Autodesk Fusion 360 part; units mm, degrees
sketch "Sketch1" plane through (0, 0, 0) normal (0, 0, 1) x (1, 0, 0)
  circle A0 centre (0, 0) radius 4
  line L0 (0, 0) -> (-60.5, 0) construction
  line L1 (-60.5, 0) -> (-121, 0) construction
  circle A1 centre (-60.5, 0) radius 3.15
  circle A2 centre (-121, 0) radius 3.15
  circle A3 centre (-60.5, 0) radius 47 construction
  circle A4 centre (-121, 0) radius 47 construction
  circle A5 centre (0, 0) radius 17.5
  circle A6 centre (-60.5, 0) radius 17 construction
  circle A7 centre (0, 0) radius 12.5 construction
  circle A8 centre (0, 30) radius 2.25
  circle A9 centre (0, -30) radius 2.25
  circle A10 centre (0, 30) radius 6 construction
  circle A11 centre (0, -30) radius 6 construction
  line L2 (-90.75, 0) -> (-90.75, 50) construction
  circle A12 centre (-90.75, 50) radius 7.5
  circle A13 centre (-90.75, 50) radius 2.25
  line L3 (-90.75, 0) -> (-90.75, -50) construction
  circle A14 centre (-90.75, -50) radius 7.5
  circle A15 centre (-90.75, -50) radius 2.25
  line L4 (-121, 0) -> (-151.25, 0) construction
  line L5 (-151.25, 0) -> (-151.25, 50) construction
  circle A16 centre (-151.25, 50) radius 7.5
  circle A17 centre (-151.25, 50) radius 2.25
  line L6 (-151.25, 0) -> (-151.25, -50) construction
  circle A18 centre (-151.25, -50) radius 7.5
  circle A19 centre (-151.25, -50) radius 2.25
  circle A20 centre (-20, 40) radius 7.5
  line L7 (-20, 40) -> (-20, 0) construction
  line L8 (-20, 0) -> (-20, -40) construction
  circle A21 centre (-20, -40) radius 7.5
  circle A22 centre (-20, -40) radius 2.25
  circle A23 centre (-20, 40) radius 2.25
  line L9 (-89.7004, -57.4262) -> (-18.9504, -47.4262)
  circle A24 centre (0, -30) radius 7.5
  circle A25 centre (0, 30) radius 7.5
  line L10 (-89.7004, 57.4262) -> (-18.9504, 47.4262)
  circle A26 centre (-196.5959, 0) radius 60
  line L11 (-16.6459, 46.7082) -> (3.3541, 36.7082)
  line L12 (7.0711, 32.5) -> (16.4992, 5.8333)
  line L13 (7.0711, -32.5) -> (16.4992, -5.8333)
  line L14 (-16.6459, -46.7082) -> (3.3541, -36.7082)
  circle A27 centre (-121, 86.6222) radius 40
  line L15 (-151.25, -57.5) -> (-90.75, -57.5)
  line L16 (-160.1233, -61.9813) -> (16.4992, -61.9813) construction
  circle A28 centre (0, 0) radius 8.5 construction
  circle A29 centre (0, 8.5) radius 1.4
  circle A30 centre (0, -8.5) radius 1.4
  line L17 (-151.25, 57.5) -> (-90.75, 57.5)
  dimension "d1" = 8
  dimension "d2" = 60.5
  dimension "d4" = 60.5
  dimension "d6" = 6.3
  dimension "d7" = 6.3
  dimension "d8" = 94
  dimension "d9" = 94
  dimension "d10" = 35
  dimension "d11" = 34
  dimension "d12" = 25
  dimension "d13" = 4.5
  dimension "d14" = 4.5
  dimension "d15" = 60
  dimension "d16" = 12
  dimension "d17" = 12
  dimension "d18" = 15
  dimension "d19" = 50
  dimension "d20" = 4.5
  dimension "d21" = 15
  dimension "d22" = 4.5
  dimension "d23" = 30.25
  dimension "d24" = 15
  dimension "d25" = 4.5
  dimension "d26" = 15
  dimension "d27" = 4.5
  dimension "d28" = 15
  dimension "d29" = 40
  dimension "d30" = 20
  dimension "d31" = 15
  dimension "d32" = 4.5
  dimension "d33" = 4.5
  dimension "d34" = 15
  dimension "d35" = 15
  dimension "d36" = 120
  dimension "d37" = 80
  dimension "d44" = 17
  dimension "d45" = 2.8
  dimension "d46" = 2.8
extrude "Extrude1" add sketch "Sketch1" along normal blind 3.175 contours A5 | A5 A12 A14 A16 A18 A20 A21 L9 A24 A25 L10 A26 L11 L12 L13 L14 A27 L15 | A25 | A24 | A20 | A21 | A12 | A14 | A18 | A16
ref_plane "WorkPlane1" through (-70.7689, 0, 3.175) normal (0, 0, 1) x (1, 0, 0)
sketch "Sketch2" plane through (0, 0, 3.175) normal (0, 0, 1) x (1, 0, 0)
  circle A0 centre (-90.75, -50) radius 2.25
  circle A1 centre (0, 30) radius 2.25
  circle A2 centre (-151.25, -50) radius 2.25
  circle A3 centre (0, -30) radius 2.25
  circle A4 centre (0, 0) radius 4
  circle A5 centre (0, 8.5) radius 1.4
  circle A6 centre (0, -8.5) radius 1.4
  circle A7 centre (-20, -40) radius 2.25
  circle A8 centre (-90.75, 50) radius 2.25
  circle A9 centre (-20, 40) radius 2.25
  circle A10 centre (-151.25, 50) radius 2.25
  circle A11 centre (-60.5, 0) radius 3.15
  circle A12 centre (-121, 0) radius 3.15
  line L0 (-151.25, -57.5) -> (-90.75, -57.5)
  arc A13 (-156.2884, -44.4444) -> (-151.25, -57.5) centre (-151.25, -50) ccw
  arc A14 (-156.2884, -44.4444) -> (-156.2884, 44.4444) centre (-196.5959, 0) ccw
  arc A15 (-151.25, 57.5) -> (-156.2884, 44.4444) centre (-151.25, 50) ccw
  line L1 (-151.25, 57.5) -> (-90.75, 57.5)
  arc A16 (-89.7004, 57.4262) -> (-90.75, 57.5) centre (-90.75, 50) ccw
  line L2 (-89.7004, 57.4262) -> (-18.9504, 47.4262)
  arc A17 (-16.6459, 46.7082) -> (-18.9504, 47.4262) centre (-20, 40) ccw
  line L3 (-16.6459, 46.7082) -> (3.3541, 36.7082)
  arc A18 (7.0711, 32.5) -> (3.3541, 36.7082) centre (0, 30) ccw
  line L4 (7.0711, 32.5) -> (16.4992, 5.8333)
  arc A19 (16.4992, -5.8333) -> (16.4992, 5.8333) centre (0, 0) ccw
  line L5 (7.0711, -32.5) -> (16.4992, -5.8333)
  arc A20 (3.3541, -36.7082) -> (7.0711, -32.5) centre (0, -30) ccw
  line L6 (-16.6459, -46.7082) -> (3.3541, -36.7082)
  arc A21 (-18.9504, -47.4262) -> (-16.6459, -46.7082) centre (-20, -40) ccw
  line L7 (-89.7004, -57.4262) -> (-18.9504, -47.4262)
  arc A22 (-90.75, -57.5) -> (-89.7004, -57.4262) centre (-90.75, -50) ccw
equation "d2 = distBetweenGears"
equation "distBetweenGears = 60.5 mm"
equation "d4 = distBetweenGears"
equation "acrylicRoundHoleSize = 6.3 mm"
equation "d6 = acrylicRoundHoleSize"
equation "d7 = acrylicRoundHoleSize"
equation "d13 = WoodScrewHoleSize"
equation "d14 = WoodScrewHoleSize"
equation "d20 = WoodScrewHoleSize"
equation "d22 = WoodScrewHoleSize"
equation "d23 = distBetweenGears / 2"
equation "d25 = WoodScrewHoleSize"
equation "d27 = WoodScrewHoleSize"
equation "d32 = WoodScrewHoleSize"
equation "d33 = WoodScrewHoleSize"
equation "WoodScrewHoleSize = 4.5 mm"
CAD build for the part. Positions are in the model's coordinates, mm. Coordinates: 2 decimals unless noted, no trailing zeros. Order: outer loops, then holes, each group sorted by start corner. A loop starts at its lowest first (then second) coordinate and runs counter-clockwise, first axis right, second up.
(1) Mould opens along X. For faces 1 (the face through (-72, 1, 0)), 2 (the face through (11.72, 19.35, 1.57)), 3 (the face through (-92.829, 57.206, 1.565)) say: released by +X, released by -X, zero draft, split by the parting line, or undercut.
Solution:
face 1: zero draft
face 2: released by +X
face 3: undercut
(2) Pin check, flat tip, straight feed: pin 1 Ø1.5 at (y, z) = (-3, 1) entering from +X. Stop position of the tip, or through.
Solution:
pin 1: stops at x = 17.35
(3) Drill centre lines: L1, parallel to Y at x = -90.75, z = 0.9; L2, parallel to Y at x = 0, z = 1.2; L3, parallel to Y at x = -19, z = 1.5. Where is each one in solid material? Low to high.
Solution:
L1: y = -57.5 to -52.25, -47.75 to 47.75, 52.25 to 57.5
L2: y = -38.39 to -32.25, -27.75 to -9.9, -7.1 to -4, 4 to 7.1, 9.9 to 27.75, 32.25 to 38.39
L3: y = -47.43 to -42.02, -37.98 to 37.98, 42.02 to 47.43
(4) Saw through at C-C, the plane x = -122. Write the cut outline in (y, z) (3 decimals), and give its area (3 significant figures).
Solution:
outline: (-57.5, 0) - (-2.987, 0) - (-2.987, 3.175) - (-57.5, 3.175) - close; (2.987, 0) - (46.635, 0) - (46.635, 3.175) - (2.987, 3.175) - close
area: 312 mm2
(5) Saw through at D-D, the plane y = 35. Write the cut outline in (x, z) (3 decimals).
Solution:
outline: (-147.862, 0) - (5.59, 0) - (5.59, 3.175) - (-147.862, 3.175) - close
(6) Saw through at B-B, the plane z = 1.35. Count the separate pieces of the cut face and the enclosed holes in it, and give its area (3 significant figures).
Solution:
separate pieces: 1
enclosed holes: 13
area: 15,700 mm2
